```python
from build123d import *


with BuildPart() as part:
    # Croquis1 → Revolución1 (revolve)
    with BuildSketch(Plane.XY):
        with BuildLine():
            Line((17.736410427, 26.5), (27.736410427, 26.5))
            Line((27.736410427, 26.5), (27.736410427, 16))
            Line((27.736410427, 16), (21.163988978, 16))
            Line((21.163988978, 16), (17.736410427, 15.639375442))
            Line((17.736410427, 15.639375442), (17.736410427, 17.310836969))
            Line((17.736410427, 17.310836969), (21.981402985, 19.98631181))
            ThreePointArc((21.981402985, 19.98631181), (22.681602121, 21.252464086), (21.986190134, 22.521251927))
            Line((21.986190134, 22.521251927), (19.450199702, 24.133015759))
            Line((19.450199702, 24.133015759), (19.450199702, 24.770374886))
            Line((19.450199702, 24.770374886), (17.736410427, 24.770374886))
            Line((17.736410427, 24.770374886), (17.736410427, 26.5))
        make_face()
    revolve(axis=Axis((54.736410427, 0, 0), (-1, 0, 0)))


solid = part.part
```
The listing builds one solid part. Answer for the finished solid, in the listing's coordinates (mm). A direction names the side the tool comes from. Round coordinates to 2 decimals unless told otherwise and drop trailing zeros. Loops run counter-clockwise (first coordinate to the right, second up) from the corner with the lowest first, then second, coordinate; pieces in that order, holes last.
1) For faces 5 (the face through (18.581, -24.746, -1.089)), 6 (the face through (17.736, -18, 18)), 7 (the face through (24.4, -3.47, 15.62)), determine the directions among +Z, -Z, +X, -X, +Y, -Y from which every point of the face is accessible in a straight line to the end or side of a thin tool.
Outcome:
face 5: -X
face 6: +Z, -Z, -X, +Y, -Y
face 7: +X
2) A cutting plane is placed at A-A on z = 0. Determine the outline of the cut face in (x, y), plus the area to 3 significant figures.
Outcome:
outline: (17.74, -26.5) - (27.74, -26.5) - (27.74, -16) - (21.16, -16) - (17.74, -15.64) - (17.74, -17.31) - (21.98, -19.99) arc R1.5 cw to (21.99, -22.52) - (19.45, -24.13) - (19.45, -24.77) - (17.74, -24.77) - close; (17.74, 15.64) - (21.16, 16) - (27.74, 16) - (27.74, 26.5) - (17.74, 26.5) - (17.74, 24.77) - (19.45, 24.77) - (19.45, 24.13) - (21.99, 22.52) arc R1.5 cw to (21.98, 19.99) - (17.74, 17.31) - close
area: 164 mm2
3) A cutting plane is placed at C-C on x = 20.5. Determine the outline of the cut face in (y, z).
Outcome:
outline: circle Ø53 at (0, 0); circle Ø38.11 at (0, 0); hole circle Ø46.93 at (0, 0); hole circle Ø31.86 at (0, 0)
4) Consider line 1 (Y direction, x = 24.5, z = 0); line 2 (Z direction, x = 19.05, y = 0). Determine where each line is inside the solid, lowest interval first.
Outcome:
line 1: y = -26.5 to -16, 16 to 26.5
line 2: z = -26.5 to -24.77, -18.14 to -15.78, 15.78 to 18.14, 24.77 to 26.5
5) For a pull along Z with two mould halves and no side action, classify faces 1 (the face through (17.736, 13, 9)), 2 (the face through (22.806, 14.246, -22.345)), 3 (the face through (19.45, -5, 24)), 4 (the face through (18, -3.79, 17.06)) as released by +Z, released by -Z, zero draft, split by the parting line, or undercut.
Outcome:
face 1: zero draft
face 2: split by the parting line
face 3: undercut
face 4: undercut
6) Given P1, Ø1, axis at x = 26, z = -2.5, coming from the -Y side; P2, Ø3, axis at x = 22.5, z = -10.5, coming from the +Y side; P3, Ø5, axis at y = 16.5, z = 7.5, coming from the -X side; P4, Ø25, axis at y = 1.5, z = -1.5, coming from the -X side, each flat-ended and moving along its own axis, determine where each tip first touches the part or whether it passes through.
Outcome:
P1: stops at y = -26.42
P2: stops at y = 24.92
P3: stops at x = 17.74
P4: passes through
